Model file for the job. Use its own axes, mm. Give positions to 0.01 mm unless a question says otherwise; leave off trailing zeros. Write each loop counter-clockwise with the first axis right and the second up, starting at its lowest first coordinate (ties: lowest second). Pieces come first, ordered by that corner, then holes. Notation, with made-up numbers: M 26.5,72 L 73.5,72 A8 cw 73.5,85 Z; hole C 12.25,43.5 d7. An arc over 180 degrees is marked long. Answer as a JSON object with one key per item and string values. Group by question number.
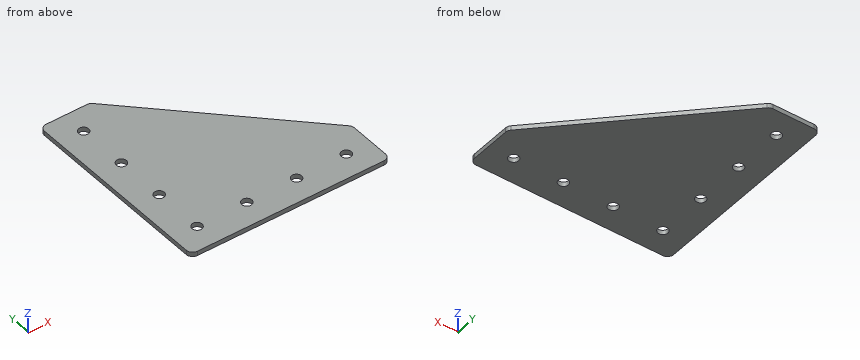
```python
from build123d import *

# Parameters (mm, degrees)
SKETCH1_R           = 2.5527
BOSS_EXTRUDE1_DEPTH = 1.143
FILLET1_R           = 3.175


with BuildPart() as part:
    # Sketch1 → Boss-Extrude1 (new, symmetric)
    with BuildSketch(Plane.XY):
        Polygon((43.046315789, -67.510526316), (43.046315789, -42.110526316), (-33.153684211, 34.089473684), (-58.553684211, 34.089473684), (-58.553684211, -67.510526316), align=None)
        with Locations((-45.853684211, 21.389473684)):
            Circle(SKETCH1_R, mode=Mode.SUBTRACT)
        with Locations((-45.853684211, -4.010526316)):
            Circle(SKETCH1_R, mode=Mode.SUBTRACT)
        with Locations((-45.853684211, -29.410526316)):
            Circle(SKETCH1_R, mode=Mode.SUBTRACT)
        with Locations((-45.853684211, -54.810526316)):
            Circle(SKETCH1_R, mode=Mode.SUBTRACT)
        with Locations((-20.453684211, -54.810526316)):
            Circle(SKETCH1_R, mode=Mode.SUBTRACT)
        with Locations((4.946315789, -54.810526316)):
            Circle(SKETCH1_R, mode=Mode.SUBTRACT)
        with Locations((30.346315789, -54.810526316)):
            Circle(SKETCH1_R, mode=Mode.SUBTRACT)
    extrude(amount=BOSS_EXTRUDE1_DEPTH, both=True)

    # Fillet1
    fillet1_edges = [part.edges().sort_by_distance(p)[0] for p in [
        (-58.553684211, 34.089473684, 0),
        (-33.153684211, 34.089473684, 0),
        (43.046315789, -42.110526316, 0),
        (43.046315789, -67.510526316, 0),
        (-58.553684211, -67.510526316, 0),
    ]]
    fillet(fillet1_edges, radius=FILLET1_R)


solid = part.part
```
Q1. Slice it at C-C, the plane x = -10. Write the cut outline in (y, z).
Q2. Drop a flat-ended pin along its axis: P1, Ø8, axis at x = -45.85, y = -4.01, coming from the -Z side. Give the stop position or say it passes through.
Q3. Slice it at A-A, the plane z = -0.8. Write the cut outline in (x, y) (3 decimals).
Q4. Wall check: L1, parallel to X at y = -56.5, z = -0.05; L2, parallel to Y at x = -46.5, z = -0.5; L3, parallel to Y at x = 7, z = -0.9. Give the ranges that are in metal, low to high.
Q5. Slice it at B-B, the plane y = -37. Write the cut outline in (x, z), then the cut area to 3 significant figures.
Solved:
{
 "1": {"outline": "M -67.51,-1.14 L 10.94,-1.14 L 10.94,1.14 L -67.51,1.14 Z"},
 "2": {"P1": "stops at z = -1.14"},
 "3": {"outline": "M -58.554,-64.336 A3.175 ccw -55.379,-67.511 L 39.871,-67.511 A3.175 ccw 43.046,-64.336 L 43.046,-43.426 A3.175 ccw 42.116,-41.181 L -32.224,33.16 A3.175 ccw -34.469,34.089 L -55.379,34.089 A3.175 ccw -58.554,30.914 Z; hole C -45.854,-54.811 d5.105; hole C -45.854,-29.411 d5.105; hole C -45.854,-4.011 d5.105; hole C -45.854,21.389 d5.105; hole C -20.454,-54.811 d5.105; hole C 4.946,-54.811 d5.105; hole C 30.346,-54.811 d5.105"},
 "4": {"L1": "x = -58.55 to -47.77, -43.94 to -22.37, -18.54 to 3.03, 6.86 to 28.43, 32.26 to 43.05", "L2": "y = -67.51 to -57.28, -52.34 to -31.88, -26.94 to -6.48, -1.54 to 18.92, 23.86 to 34.09", "L3": "y = -67.51 to -56.33, -53.29 to -6.06"},
 "5": {"outline": "M -58.55,-1.14 L 37.94,-1.14 L 37.94,1.14 L -58.55,1.14 Z", "area": "221 mm²"}
}
